For this review, take the finished solid that the model builds, in its own axes (mm). A direction names the side the tool comes from. Round coordinates to 2 decimals unless told otherwise and drop trailing zeros. Write each loop counter-clockwise with the first axis right and the second up, starting at its lowest first coordinate (ties: lowest second). Pieces come first, ordered by that corner, then holes.
from build123d import *

# Parameters (mm, degrees)
BOSS_EXTRUDE1_DEPTH                     = 60
CBORE_FOR_M5_HEX_HEAD_BOLT1_D           = 8
CBORE_FOR_M5_HEX_HEAD_BOLT1_CBORE_D     = 12
CBORE_FOR_M5_HEX_HEAD_BOLT1_CBORE_DEPTH = 10
MIRROR2_COPY_1_D                        = 8
MIRROR2_COPY_1_CBORE_D                  = 12
MIRROR2_COPY_1_CBORE_DEPTH              = 10
FILLET1_R                               = 10
FILLET2_R                               = 10


with BuildPart() as part:
    # Sketch1 → Boss-Extrude1 (new body)
    with BuildSketch(Plane.XY):
        Polygon((0, 0), (0, 20), (35, 20), (35, 53), (165, 50), (165, 20), (200, 20), (200, 0), align=None)
    extrude(amount=BOSS_EXTRUDE1_DEPTH)

    # CBORE for M5 Hex Head Bolt1 (through all)
    with Locations(Plane(origin=(0, 20, 0), x_dir=(1, 0, 0), z_dir=(0, 1, 0))):
        with Locations((12, -45)):
            cbore_for_m5_hex_head_bolt1 = CounterBoreHole(CBORE_FOR_M5_HEX_HEAD_BOLT1_D / 2, CBORE_FOR_M5_HEX_HEAD_BOLT1_CBORE_D / 2, CBORE_FOR_M5_HEX_HEAD_BOLT1_CBORE_DEPTH)

    # Mirror1: CBORE for M5 Hex Head Bolt1 across plane
    add(cbore_for_m5_hex_head_bolt1.mirror(Plane.XY.offset(30)), mode=Mode.SUBTRACT)

    # Mirror2: CBORE for M5 Hex Head Bolt1 across plane
    add(cbore_for_m5_hex_head_bolt1.mirror(Plane(origin=(100, 0, 0), x_dir=(0, 0, 1), z_dir=(1, 0, 0))), mode=Mode.SUBTRACT)

    # Mirror2 copy 1 (through all)
    with Locations(Plane(origin=(200, 20, 60), x_dir=(-1, 0, 0), z_dir=(0, 1, 0))):
        with Locations((12, -45)):
            CounterBoreHole(MIRROR2_COPY_1_D / 2, MIRROR2_COPY_1_CBORE_D / 2, MIRROR2_COPY_1_CBORE_DEPTH)

    # Fillet1
    fillet1_edges = [part.edges().sort_by_distance(p)[0] for p in [
        (165, 20, 30),
        (165, 50, 30),
        (35, 53, 30),
        (35, 20, 30),
    ]]
    fillet(fillet1_edges, radius=FILLET1_R)

    # Fillet2
    fillet2_edges = [part.edges().sort_by_distance(p)[0] for p in [
        (0, 10, 0),
        (200, 10, 0),
        (0, 10, 60),
        (200, 10, 60),
    ]]
    fillet(fillet2_edges, radius=FILLET2_R)


solid = part.part
(1) For faces 1 (the face through (194, 15, 45)), 2 (the face through (12, 20, 30)), 3 (the face through (165, 35, 30)), list the 3-axis set-ups (+Z, -Z, +X, -X, +Y, -Y) from which the entire face can be reached by the end or side of a thin tool; tool diameter is ignored.
Geometry check:
face 1: +Y
face 2: +Z, -Z, -X, +Y
face 3: +Z, -Z, +X, +Y
(2) We need section A-A, the plane y = 4. Give the boundary of the cut face in (x, z).
Geometry check:
outline: (0, 10) arc R10 ccw to (10, 0) - (190, 0) arc R10 ccw to (200, 10) - (200, 50) arc R10 ccw to (190, 60) - (10, 60) arc R10 ccw to (0, 50) - close; hole circle Ø8 at (12, 15); hole circle Ø8 at (12, 45); hole circle Ø8 at (188, 15); hole circle Ø8 at (188, 45)
(3) We need section D-D, the plane z = 23. Give the boundary of the cut face in (x, y), and give its area (3 significant figures).
Geometry check:
outline: (0, 0) - (200, 0) - (200, 20) - (175, 20) arc R10 cw to (165, 30) - (165, 40.23) arc R10 ccw to (155.23, 50.23) - (45.23, 52.76) arc R10 ccw to (35, 42.77) - (35, 30) arc R10 cw to (25, 20) - (0, 20) - close
area: 8,090 mm2
(4) Mouldability with a two-part tool opening along Z and no side actions: class faces 4 (the face through (167.85, 23.01, 30.42)), 5 (the face through (12.521, 4.93, 18.966)), 6 (the face through (189.42, 10, 11.08)), 7 (the face through (196.99, 9.86, 57.15)) as pulls with the +Z half, pulls with the -Z half, needs draft (parallel to the pull), parting line crosses it, or undercut.
Geometry check:
face 4: needs draft
face 5: undercut
face 6: undercut
face 7: pulls with the +Z half
(5) For line 1 along Z through (x, y) = (11.5, 15); line 2 along Z through (x, y) = (188, 2.25); line 3 along X through (y, z) = (18.5, 10.5), list the stretches that pass through material, from the lowest coordinate up.
Geometry check:
line 1: z = 0 to 9.02, 20.98 to 39.02, 50.98 to 60
line 2: z = 0 to 11, 19 to 41, 49 to 60
line 3: x = 0 to 8.03, 15.97 to 184.03, 191.97 to 200
(6) For pin 1 Ø10 at (y, z) = (39, 41) entering from -X; pin 2 Ø3 at (x, z) = (124.5, 34) entering from +Y; pin 3 Ø8 at (y, z) = (34.5, 24) entering from +X, all flat-tipped, find the tip position at first contact; note any pin that passes through.
Geometry check:
pin 1: stops at x = 35
pin 2: stops at y = 50.97
pin 3: stops at x = 165
(7) We need section B-B, the plane z = 15. Give the boundary of the cut face in (x, y), and give its area (3 significant figures).
Geometry check:
outline: (0, 0) - (8, 0) - (8, 10) - (6, 10) - (6, 20) - (0, 20) - close; (16, 0) - (184, 0) - (184, 10) - (182, 10) - (182, 20) - (175, 20) arc R10 cw to (165, 30) - (165, 40.23) arc R10 ccw to (155.23, 50.23) - (45.23, 52.76) arc R10 ccw to (35, 42.77) - (35, 30) arc R10 cw to (25, 20) - (18, 20) - (18, 10) - (16, 10) - close; (192, 0) - (200, 0) - (200, 20) - (194, 20) - (194, 10) - (192, 10) - close
area: 7,690 mm2
(8) We need section C-C, the plane x = 12. Give the boundary of the cut face in (y, z), and give its area (3 significant figures).
Geometry check:
outline: (0, 0) - (20, 0) - (20, 9) - (10, 9) - (10, 11) - (0, 11) - close; (0, 19) - (10, 19) - (10, 21) - (20, 21) - (20, 39) - (10, 39) - (10, 41) - (0, 41) - close; (0, 49) - (10, 49) - (10, 51) - (20, 51) - (20, 60) - (0, 60) - close
area: 800 mm2
